Here's how the part is built. I have some questions about the finished solid (model axes, mm). Round coordinates to 2 decimals unless told otherwise and drop trailing zeros. Loops run counter-clockwise (first coordinate to the right, second up) from the corner with the lowest first, then second, coordinate; pieces in that order, holes last. Notation, with made-up numbers: (15, 64.25) - (21, 64.25) arc R24 cw to (21, 85.25) - close; hole circle Ø8 at (3, 31.25). An arc over 180 degrees is marked (long way). Answer as a JSON object with one key per item and string values. Group by question number.
1) If we mould it in two halves opening along X, with no side actions, what happens to faces 1 (the face through (3, 1, 1.588)), 2 (the face through (-0.454, 6.844, -0.022)), 3 (the face through (12.7, -7, 0))? For each: pulls with the +X half, pulls with the -X half, needs draft (parallel to the pull), parting line crosses it, or undercut.
2) I want a section at B-B, the plane y = 0. Please give me the cut outline in (x, z), then the cut area to 3 significant figures.
3) If I drill on line 1 along Y through (x, z) = (0, 0); line 2 along X through (y, z) = (0, 0.2); line 3 along Y through (x, z) = (1.25, -1.2), over which ranges is the centre line in solid material (lowest first)? Write a range as [from, to].
4) Will this pin go through, and if not, where does the flat tip stop? P1, Ø2.5, axis at x = 0, y = 0, coming from the +Z side.
5) I want a section at A-A, the plane z = -0.55. Please give me the cut outline in (x, y).
6) I want a section at C-C, the plane x = 1. Please give me the cut outline in (y, z), then the cut area to 3 significant figures.
7) I want a section at D-D, the plane y = 32. Please give me the cut outline in (x, z).
from build123d import *

# Parameters (mm, degrees)
BOSS_EXTRUDE1_DEPTH     = 1.5875
CUT_EXTRUDE1_DEPTH      = 41.286233691
CUT_EXTRUDE1_DEPTH_BACK = 41.286233691
SKETCH2_R               = 2.0955


with BuildPart() as part:
    # Sketch1 → Boss-Extrude1 (new, symmetric)
    with BuildSketch(Plane.XY):
        Polygon((12.7, 25.4), (6.588707745, 38.1), (-6.588707745, 38.1), (-12.7, 25.4), (-12.7, -38.1), (12.7, -38.1), align=None)
    extrude(amount=BOSS_EXTRUDE1_DEPTH, both=True)

    # Sketch2 → Cut-Extrude1 (cut, two sides: drawn at the far end of the back side and taken through both)
    with BuildSketch(Plane.XY.offset(1.5875).offset(-CUT_EXTRUDE1_DEPTH_BACK)):
        with Locations((0, -25.4)):
            Circle(SKETCH2_R)
        Circle(SKETCH2_R)
        with Locations((0, 25.4)):
            Circle(SKETCH2_R)
        with Locations((0, -8.89)):
            Circle(SKETCH2_R)
        with Locations((0, 8.89)):
            Circle(SKETCH2_R)
    extrude(amount=CUT_EXTRUDE1_DEPTH + CUT_EXTRUDE1_DEPTH_BACK, mode=Mode.SUBTRACT)


solid = part.part
Outcome:
{
 "1": {"face 1": "needs draft", "face 2": "undercut", "face 3": "pulls with the +X half"},
 "2": {"outline": "(-12.7, -1.59) - (-2.1, -1.59) - (-2.1, 1.59) - (-12.7, 1.59) - close; (2.1, -1.59) - (12.7, -1.59) - (12.7, 1.59) - (2.1, 1.59) - close", "area": "67.3 mm^2"},
 "3": {"line 1": "[-38.1, -27.5], [-23.3, -10.99], [-6.79, -2.1], [2.1, 6.79], [10.99, 23.3], [27.5, 38.1]", "line 2": "[-12.7, -2.1], [2.1, 12.7]", "line 3": "[-38.1, -27.08], [-23.72, -10.57], [-7.21, -1.68], [1.68, 7.21], [10.57, 23.72], [27.08, 38.1]"},
 "4": {"P1": "through"},
 "5": {"outline": "(-12.7, -38.1) - (12.7, -38.1) - (12.7, 25.4) - (6.59, 38.1) - (-6.59, 38.1) - (-12.7, 25.4) - close; hole circle Ø4.19 at (0, -25.4); hole circle Ø4.19 at (0, -8.89); hole circle Ø4.19 at (0, 0); hole circle Ø4.19 at (0, 8.89); hole circle Ø4.19 at (0, 25.4)"},
 "6": {"outline": "(-38.1, -1.59) - (-27.24, -1.59) - (-27.24, 1.59) - (-38.1, 1.59) - close; (-23.56, -1.59) - (-10.73, -1.59) - (-10.73, 1.59) - (-23.56, 1.59) - close; (-7.05, -1.59) - (-1.84, -1.59) - (-1.84, 1.59) - (-7.05, 1.59) - close; (1.84, -1.59) - (7.05, -1.59) - (7.05, 1.59) - (1.84, 1.59) - close; (10.73, -1.59) - (23.56, -1.59) - (23.56, 1.59) - (10.73, 1.59) - close; (27.24, -1.59) - (38.1, -1.59) - (38.1, 1.59) - (27.24, 1.59) - close", "area": "183 mm^2"},
 "7": {"outline": "(-9.52, -1.59) - (9.52, -1.59) - (9.52, 1.59) - (-9.52, 1.59) - close"}
}
